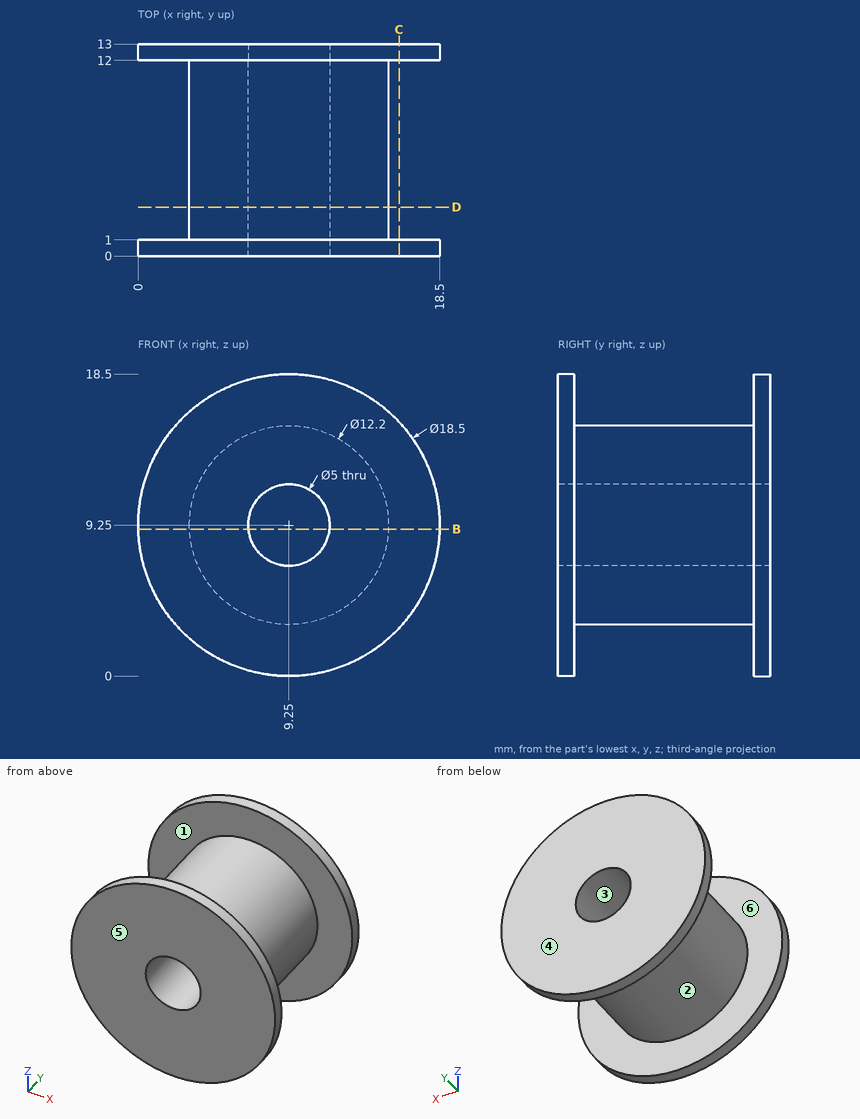
Answer from the drawing. Dimensions are ordinates in mm from the lowest x, y and z of the part. A direction names the side the tool comes from. Give positions to 0.01 mm unless a question says otherwise; leave off trailing zeros. Write each loop counter-clockwise with the first axis right and the second up, starting at its lowest first coordinate (ties: lowest second). Pieces come first, ordered by that corner, then holes. Notation, with made-up numbers: (-9.75, 82) - (29.25, 82) arc R22 cw to (29.25, 95) - close; hole circle Ø11 at (-30, 20.25). An arc over 180 degrees is marked (long way). One line per item, written item: value. Start each with the question number.
1. Find section C-C (x = 16). Write down the section's boundary in (y, z).
2. Find section D-D (y = 3). Write down the section's boundary in (x, z).
3. Consider probe 1 along Y at (x, z) = (6.75, 2.5); probe 2 along Z at (x, y) = (9.25, 8.75). Determine where each line is inside the solid, lowest interval first.
4. Find section B-B (z = 9). Write down the section's boundary in (x, y).
5. For the marked faces 5 and 6, determine the directions among +Z, -Z, +X, -X, +Y, -Y from which every point of the face is accessible in a straight line to the end or side of a thin tool.
6. Given pin 1 (5 mm diameter, centred on y = 7.5, z = 16.5, fed in from +X); pin 2 (5 mm diameter, centred on x = 14.5, z = 6.5, fed in from -Y); pin 3 (2 mm diameter, centred on y = 2.5, z = 9.5, fed in from +X); pin 4 (6 mm diameter, centred on y = 2.5, z = 3, fed in from +X), each flat-ended and moving along its own axis, determine where each tip first touches the part or whether it passes through.
7. For a pull along Y with two mould halves and no side action, classify the marked faces 1, 2, 3 and 4 as +Y half, -Y half, draft (parallel to the pull), parting line (faces both ways), or undercut.
Geometry results:
1. outline: (0, 2.93) - (1, 2.93) - (1, 15.57) - (0, 15.57) - close; (12, 2.93) - (13, 2.93) - (13, 15.57) - (12, 15.57) - close
2. outline: circle Ø12.2 at (9.25, 9.25); hole circle Ø5 at (9.25, 9.25)
3. probe 1: 0 to 1, 12 to 13
3. probe 2: 3.15 to 6.75, 11.75 to 15.35
4. outline: (0, 0) - (6.76, 0) - (6.76, 13) - (0, 13) - (0, 12) - (3.16, 12) - (3.16, 1) - (0, 1) - close; (11.74, 0) - (18.5, 0) - (18.5, 1) - (15.34, 1) - (15.34, 12) - (18.5, 12) - (18.5, 13) - (11.74, 13) - close
5. face 5: +Z, -Z, +X, -X, -Y
5. face 6: none
6. pin 1: x = 13.08
6. pin 2: y = 0
6. pin 3: x = 15.35
6. pin 4: x = 17.75
7. face 1: undercut
7. face 2: undercut
7. face 3: draft
7. face 4: +Y half
